from build123d import *

# Parameters (mm, degrees)
BASE_DEPTH                             = 3
ESQUISSE2_R                            = 3
PER_AGE_PROFIL_DEPTH                   = 5
ESQUISSE3_R                            = 2.3
PER_AGE_LIDAR_DEPTH                    = 4
ESQUISSE4_R                            = 11.25
PER_AGE_BOUTON_D_ARRET_D_URGENCE_DEPTH = 4
ESQUISSE5_R                            = 7
PER_AGE_TIRETTE_DEPTH                  = 4
PER_AGE_CABLE_MANAGEMENT_DEPTH         = 4
SKETCH1_W                              = 10
SKETCH1_H                              = 3
SKETCH1_W_2                            = 3
SKETCH1_H_2                            = 10
CUT_EXTRUDE1_DEPTH                     = 4
CONG_1_R                               = 3
ESQUISSE10_W                           = 90
ESQUISSE10_H                           = 1
ESQUISSE10_W_2                         = 1
ESQUISSE10_H_2                         = 170
ESQUISSE10_W_3                         = 110
ESQUISSE10_H_3                         = 30
BOSS_EXTRU_1_DEPTH                     = 2


with BuildPart() as part:
    # Esquisse1 → Base (new body)
    with BuildSketch(Plane.XY):
        Polygon((-99.748737342, 120), (-75, 144.748737342), (75, 144.748737342), (99.748737342, 120), (99.748737342, -120), (75, -144.748737342), (-75, -144.748737342), (-99.748737342, -120), align=None)
    extrude(amount=BASE_DEPTH)

    # Esquisse2 → Perçage profilé (cut)
    with BuildSketch(Plane.XY.offset(3)):
        with Locations((-65, 121.748737342)):
            Circle(ESQUISSE2_R)
        with Locations((65, 121.748737342)):
            Circle(ESQUISSE2_R)
        with Locations((65, -121.748737342)):
            Circle(ESQUISSE2_R)
        with Locations((-65, -121.748737342)):
            Circle(ESQUISSE2_R)
    extrude(amount=-PER_AGE_PROFIL_DEPTH, mode=Mode.SUBTRACT)

    # Esquisse3 → Perçage Lidar (cut, through all)
    with BuildSketch(Plane(origin=(0, 0, 0), x_dir=(-1, 0, 0), z_dir=(0, 0, -1))):
        with Locations((-50, 39)):
            Circle(ESQUISSE3_R)
        with Locations((11, 50)):
            Circle(ESQUISSE3_R)
        with Locations((-50, -39)):
            Circle(ESQUISSE3_R)
        with Locations((11, -50)):
            Circle(ESQUISSE3_R)
    extrude(amount=-PER_AGE_LIDAR_DEPTH, mode=Mode.SUBTRACT)

    # Esquisse4 → Perçage bouton d'arret d'urgence (cut, through all)
    with BuildSketch(Plane(origin=(0, 0, 0), x_dir=(-1, 0, 0), z_dir=(0, 0, -1))):
        with Locations((25, -109.748737342)):
            Circle(ESQUISSE4_R)
    extrude(amount=-PER_AGE_BOUTON_D_ARRET_D_URGENCE_DEPTH, mode=Mode.SUBTRACT)

    # Esquisse5 → Perçage tirette (cut, through all)
    with BuildSketch(Plane(origin=(0, 0, 0), x_dir=(-1, 0, 0), z_dir=(0, 0, -1))):
        with Locations((-25, -109.748737342)):
            Circle(ESQUISSE5_R)
    extrude(amount=-PER_AGE_TIRETTE_DEPTH, mode=Mode.SUBTRACT)

    # Esquisse7 → Perçage cable management (cut, through all)
    with BuildSketch(Plane(origin=(0, 0, 0), x_dir=(-1, 0, 0), z_dir=(0, 0, -1))):
        with BuildLine():
            Line((-85, 7.5), (-85, -7.5))
            ThreePointArc((-85, -7.5), (-90, -12.5), (-95, -7.5))
            Line((-95, -7.5), (-95, 7.5))
            ThreePointArc((-95, 7.5), (-90, 12.5), (-85, 7.5))
        make_face()
    extrude(amount=-PER_AGE_CABLE_MANAGEMENT_DEPTH, mode=Mode.SUBTRACT)

    # Sketch1 → Cut-Extrude1 (cut, through all)
    with BuildSketch(Plane(origin=(0, 0, 0), x_dir=(-1, 0, 0), z_dir=(0, 0, -1))):
        with Locations((-40, 121.748737342)):
            Rectangle(SKETCH1_W, SKETCH1_H)
        with Locations((-20, 121.748737342)):
            Rectangle(SKETCH1_W, SKETCH1_H)
        with Locations((0, 121.748737342)):
            Rectangle(SKETCH1_W, SKETCH1_H)
        with Locations((20, 121.748737342)):
            Rectangle(SKETCH1_W, SKETCH1_H)
        with Locations((40, 121.748737342)):
            Rectangle(SKETCH1_W, SKETCH1_H)
        with Locations((-66.5, -101.748737342)):
            Rectangle(SKETCH1_W_2, SKETCH1_H_2)
        with Locations((-38.5, 85.248737342)):
            Rectangle(SKETCH1_W_2, SKETCH1_H_2)
        with Locations((-38.5, 105.248737342)):
            Rectangle(SKETCH1_W_2, SKETCH1_H_2)
        with Locations((-66.5, -81.748737342)):
            Rectangle(SKETCH1_W_2, SKETCH1_H_2)
        with Locations((66.5, -81.748737342)):
            Rectangle(SKETCH1_W_2, SKETCH1_H_2)
        with Locations((66.5, -101.748737342)):
            Rectangle(SKETCH1_W_2, SKETCH1_H_2)
        with Locations((-30, -75.248737342)):
            Rectangle(SKETCH1_W, SKETCH1_H)
        with Locations((-50, -75.248737342)):
            Rectangle(SKETCH1_W, SKETCH1_H)
        with Locations((-10, -75.248737342)):
            Rectangle(SKETCH1_W, SKETCH1_H)
        with Locations((10, -75.248737342)):
            Rectangle(SKETCH1_W, SKETCH1_H)
        with Locations((30, -75.248737342)):
            Rectangle(SKETCH1_W, SKETCH1_H)
        with Locations((50, -75.248737342)):
            Rectangle(SKETCH1_W, SKETCH1_H)
        with Locations((-38.5, 65.248737342)):
            Rectangle(SKETCH1_W_2, SKETCH1_H_2)
        with Locations((-38.5, 45.248737342)):
            Rectangle(SKETCH1_W_2, SKETCH1_H_2)
        with Locations((-38.5, 25.248737342)):
            Rectangle(SKETCH1_W_2, SKETCH1_H_2)
        with Locations((-38.5, 5.248737342)):
            Rectangle(SKETCH1_W_2, SKETCH1_H_2)
        with Locations((-38.5, -14.751262658)):
            Rectangle(SKETCH1_W_2, SKETCH1_H_2)
        with Locations((-38.5, -34.751262658)):
            Rectangle(SKETCH1_W_2, SKETCH1_H_2)
        with Locations((-38.5, -54.751262658)):
            Rectangle(SKETCH1_W_2, SKETCH1_H_2)
    extrude(amount=-CUT_EXTRUDE1_DEPTH, mode=Mode.SUBTRACT)

    # Congé1
    cong_1_edges = [part.edges().sort_by_distance(p)[0] for p in [
        (-99.748737342, 120, 1.5),
        (-75, 144.748737342, 1.5),
        (75, 144.748737342, 1.5),
        (99.748737342, 120, 1.5),
        (99.748737342, -120, 1.5),
        (75, -144.748737342, 1.5),
        (-75, -144.748737342, 1.5),
        (-99.748737342, -120, 1.5),
    ]]
    fillet(cong_1_edges, radius=CONG_1_R)

    # Esquisse10 → Boss.-Extru.1 (add)
    with BuildSketch(Plane(origin=(0, 0, 0), x_dir=(-1, 0, 0), z_dir=(0, 0, -1))):
        with Locations((0, 120.748737342)):
            Rectangle(ESQUISSE10_W, ESQUISSE10_H)
        with Locations((-37.5, 25.248737342)):
            Rectangle(ESQUISSE10_W_2, ESQUISSE10_H_2)
        with Locations((0, -76.248737342)):
            Rectangle(ESQUISSE10_W_3, ESQUISSE10_H)
        with Locations((65.5, -91.748737342)):
            Rectangle(ESQUISSE10_W_2, ESQUISSE10_H_3)
        with Locations((-65.5, -91.748737342)):
            Rectangle(ESQUISSE10_W_2, ESQUISSE10_H_3)
    extrude(amount=-BOSS_EXTRU_1_DEPTH)


solid = part.part
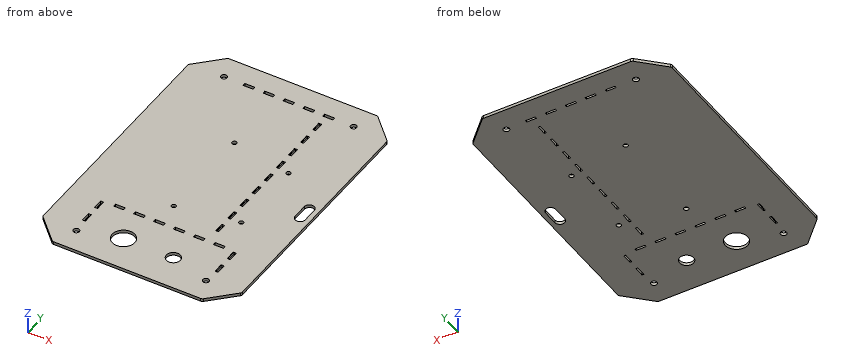
Work out the finished part from the listing and answer in its coordinate system (mm). Round coordinates to 2 decimals unless told otherwise and drop trailing zeros. Write each loop counter-clockwise with the first axis right and the second up, starting at its lowest first coordinate (ties: lowest second). Pieces come first, ordered by that corner, then holes. Notation, with made-up numbers: M 59.5,39.5 L 94.5,39.5 A23 cw 94.5,63.5 Z; hole C -12.75,37.5 d6. An arc over 180 degrees is marked long. Use a Markdown table: item, result.
1) The part is cut by section A-A on z = 0.8. State how many separate pieces and enclosed holes the cut face has, plus the area to 3 significant figures.
Taken from the geometry:
| item | result |
|---|---|
| separate pieces | 1 |
| enclosed holes | 35 |
| area | 55,100 mm2 |
2) The part is cut by section B-B on x = -80.5. Give the vertices of the cut face in (y, z), plus the area to 3 significant figures.
Taken from the geometry:
| item | result |
|---|---|
| outline | M -139.25,0 L 139.25,0 L 139.25,3 L -139.25,3 Z |
| area | 835 mm2 |
3) Consider line 1 (X direction, y = -84, z = 1.95); line 2 (X direction, y = -97, z = 2.2); line 3 (Y direction, x = 50, z = 0.8). Determine where each line is inside the solid, lowest interval first. Write a range as [from, to].
Taken from the geometry:
| item | result |
|---|---|
| line 1 | x = [-99.75, -68], [-66, 66], [68, 99.75] |
| line 2 | x = [-99.75, -68], [-65, 65], [68, 99.75] |
| line 3 | y = [-144.75, -75.75], [-73.75, -41.3], [-36.7, 36.7], [41.3, 144.75] |
4) A flat-ended cylindrical pin translates along its axis: pin 1 (0.8 mm diameter, centred on x = 37.5, y = 27, fed in from +Z). Find the tip coordinate at first contact, or state that the pin passes through.
Taken from the geometry:
| item | result |
|---|---|
| pin 1 | stops at z = 2 |
